Model file for the job. Use its own axes, mm. A direction names the side the tool comes from. Round coordinates to 2 decimals unless told otherwise and drop trailing zeros. Order: outer loops, then holes, each group sorted by start corner. A loop starts at its lowest first (then second) coordinate and runs counter-clockwise, first axis right, second up. Notation, with made-up numbers: (37, -24.75) -> (61, -24.75) arc R15 ccw to (61, -2.75) -> close; hole circle Ø7 at (-34.75, 0). An arc over 180 degrees is marked (long way). Use CSV: the item, a comma, the result in double quotes.
```python
from build123d import *

# Parameters (mm, degrees)
F0_R         = 32.258
F0_R_2       = 3.6322
F1_DEPTH     = 3.175
F4_DEPTH     = 3.4925
F5_W         = 2.54
F5_H         = 20.32
F6_DEPTH     = 25.4
F7_R         = 1.26999
F8_R         = 3.4798
F9_R         = 32.258
F9_R_2       = 31.242
F10_DEPTH    = 7.62
F12_DEPTH    = 1.5748
F13_T1_DEPTH = 3.175
F13_T3_DEPTH = 1.5748
F14_R        = 2.5029708097
F15_DEPTH    = 0.762
F16_T1_DEPTH = 0.762
F17_R        = 1.016
F18_DEPTH    = 25.4
F19_R        = 1.5875
F20_DEPTH    = 1.524


# Not quite as in the source:
# - a fillet or chamfer that OpenCascade refuses, or shapes differently, is made with other operations: its cross-section is extruded or revolved along the edge and cut away or added
# - a fillet or chamfer is up to 0.001 mm smaller than in the source, because OpenCascade refuses the exact size


with BuildPart() as f1:
    # F0 (on Top) → F1 (new body)
    with BuildSketch(Plane.XY):
        Circle(F0_R)
        with BuildLine():
            ThreePointArc((27.6984583499, -14.4519192165), (0, -31.242), (-27.6984583499, -14.4519192165))
            Line((-27.6984583499, -14.4519192165), (-23.1550479516, -11.82878))
            Line((-23.1550479516, -11.82878), (23.1550479516, -11.82878))
            Line((23.1550479516, -11.82878), (27.6984583499, -14.4519192165))
        make_face(mode=Mode.SUBTRACT)
        with BuildLine():
            ThreePointArc((-1.5875, 4.2197649224), (-1.9273330318, 4.0757771817), (-2.25425, 3.904475533))
            Line((-2.25425, 3.904475533), (-29.0274080844, -11.5530144941))
            ThreePointArc((-29.0274080844, -11.5530144941), (-26.2927422142, 16.8746635777), (-1.5875, 31.2016411067))
            Line((-1.5875, 31.2016411067), (-1.5875, 4.2197649224))
        make_face(mode=Mode.SUBTRACT)
        Circle(F0_R_2, mode=Mode.SUBTRACT)
        with BuildLine():
            Line((29.0274080844, -11.5530144941), (2.25425, 3.904475533))
            ThreePointArc((2.25425, 3.904475533), (1.9273330318, 4.0757771817), (1.5875, 4.2197649224))
            Line((1.5875, 4.2197649224), (1.5875, 31.2016411067))
            ThreePointArc((1.5875, 31.2016411067), (26.2927422142, 16.8746635777), (29.0274080844, -11.5530144941))
        make_face(mode=Mode.SUBTRACT)
    extrude(amount=-F1_DEPTH)

    # F3 (on offset) → F4 (join, symmetric)
    with BuildSketch(Plane.YZ):
        with BuildLine():
            ThreePointArc((0, -26.9952715967), (-14.4117945702, -18.019693004), (-6.1718963048, -3.175))
            Line((-6.1718963048, -3.175), (-6.1718963048, -2.7284894604))
            Line((-6.1718963048, -2.7284894604), (-11.8285217471, -2.7284894604))
            ThreePointArc((-11.8285217471, -2.7284894604), (-17.8532575218, -14.8291637745), (-11.9875892757, -27.0077390621))
            ThreePointArc((-11.9875892757, -27.0077390621), (-10.1388723772, -28.0174760831), (-8.0615554064, -28.3668715967))
            Line((-8.0615554064, -28.3668715967), (3.7295622751, -28.3668715967))
            Line((3.7295622751, -28.3668715967), (3.7295622751, -26.9952715967))
            Line((3.7295622751, -26.9952715967), (0, -26.9952715967))
        make_face()
    extrude(amount=F4_DEPTH, both=True)

    # F5 (on Front) → F6 (cut)
    with BuildSketch(Plane.XZ):
        with Locations((0, -14.732)):
            Rectangle(F5_W, F5_H)
    extrude(amount=F6_DEPTH, mode=Mode.SUBTRACT)

    # F7 (radius 1.27 in the source; OpenCascade refuses exactly that, so slightly less here)
    f7_edges = [f1.edges().sort_by_distance(p)[0] for p in [
        (1.27, -11.496811, -4.572),
        (-1.27, -11.496811, -4.572),
        (1.27, -11.960099, -24.892),
        (-1.27, -11.960099, -24.892),
    ]]
    fillet(f7_edges, radius=F7_R)

    # F8
    f8_edges = [f1.edges().sort_by_distance(p)[0] for p in [
        (-3.4925, 3.729562, -27.681072),
        (3.4925, 3.729562, -27.681072),
    ]]
    fillet(f8_edges, radius=F8_R)

    # F9 (on face) → F10 (join)
    with BuildSketch(Plane.XY):
        Circle(F9_R)
        Circle(F9_R_2, mode=Mode.SUBTRACT)
    extrude(amount=F10_DEPTH)

    # F11 (on face) → F12 (cut)
    with BuildSketch(Plane.XY):
        with BuildLine():
            Line((-6.35, -2.1263810414), (-23.1550479516, -11.82878))
            Line((-23.1550479516, -11.82878), (-23.1550479516, -13.7292239815))
            Line((-23.1550479516, -13.7292239815), (23.1550479516, -13.8936461881))
            Line((23.1550479516, -13.8936461881), (23.1550479516, -11.82878))
            Line((23.1550479516, -11.82878), (6.35, -2.1263810414))
            ThreePointArc((6.35, -2.1263810414), (0, -6.6965660105), (-6.35, -2.1263810414))
        make_face()
    extrude(amount=-F12_DEPTH, mode=Mode.SUBTRACT)

    # F13: fillet of radius 5.08 on 10 edges, made by hand

    # F13_s2 → F13_t1 (join)
    with BuildSketch(Plane.XY.offset(-3.175)):
        with BuildLine():
            ThreePointArc((1.5875, 7.2223631924), (2.2680909488, 4.6823631924), (4.1275, 2.8229541412))
            Line((4.1275, 2.8229541412), (3.8735, 2.3830132361))
            ThreePointArc((3.8735, 2.3830132361), (2.00025, 3.4645346278), (1.4086267606, 3.7442984522))
            Line((1.4086267606, 3.7442984522), (1.0795, 4.2197649224))
            Line((1.0795, 4.2197649224), (1.0795, 7.2223631924))
            Line((1.0795, 7.2223631924), (1.5875, 7.2223631924))
        make_face()
        with BuildLine():
            ThreePointArc((-4.1275, 2.8229541412), (-2.2680909488, 4.6823631924), (-1.5875, 7.2223631924))
            Line((-1.5875, 7.2223631924), (-1.0795, 7.2223631924))
            Line((-1.0795, 7.2223631924), (-1.0795, 4.2197649224))
            Line((-1.0795, 4.2197649224), (-1.4086267606, 3.7442984522))
            ThreePointArc((-1.4086267606, 3.7442984522), (-2.00025, 3.4645346278), (-3.8735, 2.3830132361))
            Line((-3.8735, 2.3830132361), (-4.1275, 2.8229541412))
        make_face()
        with BuildLine():
            ThreePointArc((1.5875, 25.2981162886), (3.5667318521, 29.3219995987), (7.9621601942, 30.2103718786))
            ThreePointArc((7.9621601942, 30.2103718786), (4.8004849887, 30.870988126), (1.5875, 31.2016411067))
            Line((1.5875, 31.2016411067), (1.5875, 25.2981162886))
        make_face()
        with BuildLine():
            ThreePointArc((-7.9621601942, 30.2103718786), (-3.5667318521, 29.3219995987), (-1.5875, 25.2981162886))
            Line((-1.5875, 25.2981162886), (-1.5875, 31.2016411067))
            ThreePointArc((-1.5875, 31.2016411067), (-4.8004849887, 30.870988126), (-7.9621601942, 30.2103718786))
        make_face()
        with BuildLine():
            ThreePointArc((-23.0901860951, -11.7913319897), (-25.5388151591, -15.2315851298), (-24.5405134922, -19.3345742528))
            ThreePointArc((-24.5405134922, -19.3345742528), (-26.2333304182, -16.9668777083), (-27.6984583499, -14.4519192165))
            Line((-27.6984583499, -14.4519192165), (-23.0901860951, -11.7913319897))
        make_face()
        with BuildLine():
            ThreePointArc((-23.3346480943, -8.2662979814), (-28.0816389218, -8.4424316835), (-30.8988516077, -4.6177411496))
            ThreePointArc((-30.8988516077, -4.6177411496), (-30.1631174493, -8.1393433235), (-29.0274080844, -11.5530144941))
            Line((-29.0274080844, -11.5530144941), (-23.3346480943, -8.2662979814))
        make_face()
        with BuildLine():
            ThreePointArc((24.5405134922, -19.3345742528), (25.5388151591, -15.2315851298), (23.0901860951, -11.7913319897))
            Line((23.0901860951, -11.7913319897), (27.6984583499, -14.4519192165))
            ThreePointArc((27.6984583499, -14.4519192165), (26.2333304182, -16.9668777083), (24.5405134922, -19.3345742528))
        make_face()
        with BuildLine():
            ThreePointArc((30.8988516077, -4.6177411496), (28.0816389218, -8.4424316835), (23.3346480943, -8.2662979814))
            Line((23.3346480943, -8.2662979814), (29.0274080844, -11.5530144941))
            ThreePointArc((29.0274080844, -11.5530144941), (30.1631174493, -8.1393433235), (30.8988516077, -4.6177411496))
        make_face()
    extrude(amount=F13_T1_DEPTH)

    # F13_s4 → F13_t3 (join)
    with BuildSketch(Plane.XY.offset(-1.5748)):
        with BuildLine():
            ThreePointArc((4.4329020877, -5.0193002913), (7.2889409664, -3.7722686868), (10.3356916982, -4.4275212163))
            Line((10.3356916982, -4.4275212163), (6.35, -2.1263810414))
            ThreePointArc((6.35, -2.1263810414), (5.5821133816, -3.6991899827), (4.4329020877, -5.0193002913))
        make_face()
        with BuildLine():
            ThreePointArc((-10.3356916982, -4.4275212163), (-7.2889409664, -3.7722686868), (-4.4329020877, -5.0193002913))
            ThreePointArc((-4.4329020877, -5.0193002913), (-5.5821133816, -3.6991899827), (-6.35, -2.1263810414))
            Line((-6.35, -2.1263810414), (-10.3356916982, -4.4275212163))
        make_face()
    extrude(amount=F13_T3_DEPTH)

    # F14 (on face) → F15 (join)
    with BuildSketch(Plane.XY.offset(-1.5748)):
        with Locations((0, -7.0612)):
            Circle(F14_R)
    extrude(amount=F15_DEPTH)

    # F16: fillet of radius 5.08 on 2 edges, made by hand

    # F16_s2 → F16_t1 (join)
    with BuildSketch(Plane.XY.offset(-1.5748)):
        with BuildLine():
            ThreePointArc((-4.123339334, -5.2765584494), (-3.0648098759, -6.4018902356), (-2.3934920763, -7.7933601976))
            ThreePointArc((-2.3934920763, -7.7933601976), (-2.5027259003, -7.02618654), (-2.3720733098, -6.2623689245))
            ThreePointArc((-2.3720733098, -6.2623689245), (-3.2848975519, -5.8355329154), (-4.123339334, -5.2765584494))
        make_face()
        with BuildLine():
            ThreePointArc((4.123339334, -5.2765584494), (3.0648098759, -6.4018902356), (2.3934920763, -7.7933601976))
            ThreePointArc((2.3934920763, -7.7933601976), (2.5027259003, -7.02618654), (2.3720733098, -6.2623689245))
            ThreePointArc((2.3720733098, -6.2623689245), (3.2848975519, -5.8355329154), (4.123339334, -5.2765584494))
        make_face()
    extrude(amount=F16_T1_DEPTH)

    # F17 (on face) → F18 (cut)
    with BuildSketch(Plane.XY):
        with Locations((0, -7.0612)):
            Circle(F17_R)
    extrude(amount=-F18_DEPTH, mode=Mode.SUBTRACT)

    # F19 (on face) → F20 (cut)
    with BuildSketch(Plane.XY):
        with Locations((0, -7.0612)):
            Circle(F19_R)
    extrude(amount=-F20_DEPTH, mode=Mode.SUBTRACT)


solid = f1.part
```
Q1. Probe line 1 along Y through (x, z) = (0, -1.8); line 2 along Y through (x, z) = (0, -3); line 3 along Z through (x, y) = (-5, 2) (3 decimals). List the from-to ranges inside material, lowest first.
From the geometry:
line 1,"y = -32.26 to -31.24, -11.83 to -8.08, -6.05 to -3.63, 3.63 to 32.26"
line 2,"y = -32.26 to -31.24, -12.17 to -8.08, -6.05 to -3.63, 3.63 to 32.26"
line 3,"z = -3.175 to 0"
Q2. Cut at A-A (x = -5.5). Give the cut face in (y, z) (3 decimals), plus the area to 3 significant figures.
From the geometry:
outline,"(-31.786, -3.175) -> (-30.754, -3.175) -> (-30.754, 7.62) -> (-31.786, 7.62) -> close; (-11.829, -3.175) -> (2.031, -3.175) -> (2.031, 0) -> (-4.295, 0) -> (-4.295, -1.575) -> (-11.829, -1.575) -> close; (30.242, -3.175) -> (31.786, -3.175) -> (31.786, 7.62) -> (30.754, 7.62) -> (30.754, 0) -> (30.242, 0) -> close"
area,"56.0 mm²"
Q3. Cut at D-D (y = 22.5). Give the cut face in (x, z) (1 decimal).
From the geometry:
outline,"(-23.1, -3.2) -> (-21.7, -3.2) -> (-21.7, 7.6) -> (-23.1, 7.6) -> close; (-1.6, -3.2) -> (1.6, -3.2) -> (1.6, 0) -> (-1.6, 0) -> close; (21.7, -3.2) -> (23.1, -3.2) -> (23.1, 7.6) -> (21.7, 7.6) -> close"
Q4. Mould opens along Z. For faces 3 (the flat face through (-1.27, -15, -15)), 4 (the flat face through (-13.597, -2.644, -1.565)), 5 (the cylindrical face through (1.6, -17.85, -14.63)) say: +Z half, -Z half, draft (parallel to the pull), parting line (faces both ways), or undercut.
From the geometry:
face 3,"undercut"
face 4,"draft"
face 5,"parting line"
Q5. Cut at C-C (y = -1.5). Give the cut face in (x, z) (1 decimal), plus the area to 3 significant figures.
From the geometry:
outline,"(-32.2, -3.2) -> (-31.2, -3.2) -> (-31.2, 7.6) -> (-32.2, 7.6) -> close; (-11.6, -3.2) -> (-3.3, -3.2) -> (-3.3, 0) -> (-11.6, 0) -> close; (-3.5, -28.4) -> (3.5, -28.4) -> (3.5, -27.2) -> (-3.5, -27.2) -> close; (3.3, -3.2) -> (11.6, -3.2) -> (11.6, 0) -> (3.3, 0) -> close; (31.2, -3.2) -> (32.2, -3.2) -> (32.2, 7.6) -> (31.2, 7.6) -> close"
area,"82.8 mm²"
Q6. Which spindle directions (+Z, -Z, +X, -X, +Y, -Y) get a long thin tool onto all of the face, cutting with end or side? Do faces 1 (the cylindrical face through (25.55, -15.29, -1.61)), 2 (the cylindrical face through (3.08, -6.38, -1.2)). Say none if no direction does.
From the geometry:
face 1,"+Z, -Z"
face 2,"+Z"
Q7. Cut at B-B (z = -21.5). Give the cut face in (x, y).
From the geometry:
outline,"(-3.49, -16.38) -> (-1.27, -16.38) -> (-1.27, -12.91) -> (-3.49, -12.91) -> close; (1.27, -16.38) -> (3.49, -16.38) -> (3.49, -12.91) -> (1.27, -12.91) -> close"
Q8. Pin check, flat tips, straight feed: pin 1 (2.5 mm diameter, centred on y = 17, z = -2, fed in from +X); pin 2 (9 mm diameter, centred on y = -8.5, z = -20, fed in from -X); pin 3 (2 mm diameter, centred on x = -7, y = -3, fed in from -Z) (3 decimals). Stop position of each tip, or through.
From the geometry:
pin 1,"stops at x = 28.15"
pin 2,"stops at x = -3.49"
pin 3,"stops at z = -3.175"
